```python
from build123d import *

# Parameters (mm, degrees)
SKETCH_1_W          = 120
SKETCH_1_H          = 10
SKETCH_1_R          = 1.5
EXTRUDE_1_DEPTH     = 10
SKETCH_2_W          = 8
SKETCH_2_H          = 8
CUT_EXTRUDE_1_DEPTH = 120


with BuildPart() as part:
    # 草图1 → 凸台-拉伸1 (new body)
    with BuildSketch(Plane(origin=(0, 0, 0), x_dir=(0, 0, -1), z_dir=(1, 0, 0))):
        with Locations((13.354414341, 5)):
            Rectangle(SKETCH_1_W, SKETCH_1_H)
        with Locations((-36.645585659, 5)):
            Circle(SKETCH_1_R, mode=Mode.SUBTRACT)
        with Locations((-26.645585659, 5)):
            Circle(SKETCH_1_R, mode=Mode.SUBTRACT)
        with Locations((58.354414341, 5)):
            Circle(SKETCH_1_R, mode=Mode.SUBTRACT)
        with Locations((48.354414341, 5)):
            Circle(SKETCH_1_R, mode=Mode.SUBTRACT)
        with Locations((38.354414341, 5)):
            Circle(SKETCH_1_R, mode=Mode.SUBTRACT)
    extrude(amount=EXTRUDE_1_DEPTH)

    # 草图2 → 切除-拉伸1 (cut)
    with BuildSketch(Plane(origin=(0, 0, -73.354414341), x_dir=(-1, 0, 0), z_dir=(0, 0, -1))):
        with Locations((-5, 5)):
            Rectangle(SKETCH_2_W, SKETCH_2_H)
    extrude(amount=-CUT_EXTRUDE_1_DEPTH, mode=Mode.SUBTRACT)


solid = part.part
```
Input: part model. Units: mm. Frame: model coordinates. A direction names the side the tool comes from. Round coordinates to 2 decimals unless told otherwise and drop trailing zeros. Loops run counter-clockwise (first coordinate to the right, second up) from the corner with the lowest first, then second, coordinate; pieces in that order, holes last. Notation, with made-up numbers: (3.25, 13) - (22.25, 13) arc R17 ccw to (22.25, 20) - close; hole circle Ø2 at (17, -10). An arc over 180 degrees is marked (long way). One line per item, written item: value. Start each with the question number.
(1) Access query for faces 4 (the cylindrical face through (0.493, 5.066, 28.144)), 5 (the flat face through (1, 5, -14)). Directions: +Z, -Z, +X, -X, +Y, -Y. A direction counts if a zero-diameter tool reaches every point of the face in a straight line with its end or side. Return the directions, or none.
(2) Ray query, line 1 (Z direction, x = 9.7, y = 5); line 2 (Y direction, x = 8.5, z = -2). Return the intervals inside material, ascending. Write a range as [from, to].
(3) Section A-A, the plane x = 3.5. Return loops of the section in (y, z), plus the area to 3 significant figures.
(4) Contact query for a flat-ended pin moving along its axis: P1, Ø3.5, axis at y = 5, z = 36.65, coming from the +X side. Output: stop coordinate, or through.
(5) Section B-B, the plane z = 21. Return loops of the section in (x, y).
(6) Draft query along X for faces 1 (the flat face through (0, 5, -13)), 2 (the flat face through (5, 1, -14)), 3 (the flat face through (5, 10, -13)). Return one class per face: +X half, -X half, draft (parallel to the pull), parting line (faces both ways), or undercut.
(7) Section C-C, the plane y = 5. Count the separate pieces of the cut face and the enclosed holes in it, plus the area to 3 significant figures.
Results below:
1. face 4: +X, -X
1. face 5: +Z, -Z
2. line 1: [-73.35, -59.85], [-56.85, -49.85], [-46.85, -39.85], [-36.85, 25.15], [28.15, 35.15], [38.15, 46.65]
2. line 2: [0, 1], [9, 10]
3. outline: (0, -73.35) - (1, -73.35) - (1, 46.65) - (0, 46.65) - close; (9, -73.35) - (10, -73.35) - (10, 46.65) - (9, 46.65) - close
3. area: 240 mm^2
4. P1: x = 10
5. outline: (0, 0) - (10, 0) - (10, 10) - (0, 10) - close; hole (1, 1) - (9, 1) - (9, 9) - (1, 9) - close
6. face 1: -X half
6. face 2: undercut
6. face 3: draft
7. separate pieces: 12
7. enclosed holes: 0
7. area: 210 mm^2
